Design review of the part built by this model. Coordinates are the model's own, in mm. A direction names the side the tool comes from. Coordinates: 2 decimals unless noted, no trailing zeros. Write each loop counter-clockwise with the first axis right and the second up, starting at its lowest first coordinate (ties: lowest second). Pieces come first, ordered by that corner, then holes. Notation, with made-up numbers: M 66.25,34 L 74.25,34 A19 cw 74.25,53 Z; hole C 83,15.25 d9. An arc over 180 degrees is marked long. Return JSON: item names as keys, results as strings. Group by question number.
```python
from build123d import *

# Parameters (mm, degrees)
F1_DEPTH      = 14
F3_START      = 2
F3_DEPTH      = 9.7
F4_DEPTH      = 1
F4_DEPTH_BACK = 22
F5_START      = 9.5
F5_DEPTH      = 4.5
F6_DEPTH      = 4.5
F8_DEPTH      = 0.5
F9_R          = 1.5933809512
F10_R         = 0.5311269837
F11_T1_DEPTH  = 5.3949137803
F11_T6_ANGLE  = 200.7294916834
F11_T12_ANGLE = 200.7294916834
F12_T1_DEPTH  = 1.2663530932
F12_T3_DEPTH  = 0.9362653772
F12_T5_DEPTH  = 1.4443499817
F12_T7_DEPTH  = 1.4443499817
F12_T9_DEPTH  = 0.9362653772
F12_T11_DEPTH = 1.2663530932
F12_T13_DEPTH = 16.1666666667
F12_T15_DEPTH = 16.1666666667
F12_T17_DEPTH = 15.3725307543
F12_T19_DEPTH = 16.3886999634
F12_T21_DEPTH = 16.3886999634
F12_T23_DEPTH = 15.3725307543
F13_SIZE      = 0.25


# Not quite as in the source:
# - a fillet or chamfer that OpenCascade refuses, or shapes differently, is made with other operations: its cross-section is extruded or revolved along the edge and cut away or added


with BuildPart() as f1:
    # F0 (on Top) → F1 (new body)
    with BuildSketch(Plane.XY):
        Polygon((6.25, 4.4), (0, 4.4), (-6.25, 4.4), (-7.5, 0), (-5.25, -5.4), (-4.395, -5.4), (-4.395, -3.9), (-2.695, -3.9), (-2.695, 0.6), (0, 0.6), (2.695, 0.6), (2.695, -3.9), (4.395, -3.9), (4.395, -5.4), (5.25, -5.4), (7.5, 0), align=None)
    extrude(amount=F1_DEPTH)

    # F2 (on Front) → F3 (cut)
    with BuildSketch(Plane.XZ.offset(F3_START)):
        Polygon((0, 4), (3.875, 4), (3.875, 9), (0, 9), (-3.875, 9), (-3.875, 4), align=None)
    extrude(amount=F3_DEPTH, mode=Mode.SUBTRACT)

    # F2 (on Front) → F4 (cut, two sides)
    with BuildSketch(Plane.XZ) as f4_sk:
        Polygon((-3.875, 1), (0, 1), (3.875, 1), (3.875, 4), (0, 4), (-3.875, 4), align=None)
    extrude(amount=-F4_DEPTH, mode=Mode.SUBTRACT)
    extrude(f4_sk.sketch, amount=F4_DEPTH_BACK, mode=Mode.SUBTRACT)

    # F0 (on Top) → F5 (join)
    with BuildSketch(Plane.XY.offset(F5_START)):
        Polygon((0, -5.4), (4.395, -5.4), (4.395, -3.9), (2.695, -3.9), (2.695, 0.6), (0, 0.6), (-2.695, 0.6), (-2.695, -3.9), (-4.395, -3.9), (-4.395, -5.4), align=None)
    extrude(amount=F5_DEPTH)

    # F6 (add): a face of the model
    f6_faces = [f1.faces().sort_by_distance(p)[0] for p in [
        (0, 0.6, 6.75),
    ]]
    extrude(f6_faces, amount=F6_DEPTH)

    # F7 (on face) → F8 (join)
    with BuildSketch(Plane(origin=(0, 0, 0), x_dir=(1, 0, 0), z_dir=(0, 0, -1))):
        Polygon((4.395, 5.4), (4.395, 4.4), (4.5833333333, 4.4), (6.4426875763, -0.062450183), (5.4945200146, -3.4), (-5.4945200146, -3.4), (-6.4426875763, -0.062450183), (-4.5833333333, 4.4), (-4.395, 4.4), (-4.395, 5.4), (-5.25, 5.4), (-7.5, 0), (-6.25, -4.4), (6.25, -4.4), (7.5, 0), (5.25, 5.4), align=None)
    extrude(amount=F8_DEPTH)

    # F9
    f9_edges = [f1.edges().sort_by_distance(p)[0] for p in [
        (2.695, 0.6, 0.5),
        (-2.695, 0.6, 0.5),
    ]]
    fillet(f9_edges, radius=F9_R)

    # F10
    f10_edges = [f1.edges().sort_by_distance(p)[0] for p in [
        (-3.285, -3.9, 1),
        (3.285, -3.9, 1),
    ]]
    fillet(f10_edges, radius=F10_R)

    # F11: fillet of radius 0.4104163056 on 2 edges, made by hand

    # F11_s2 → F11_t1 (join)
    with BuildSketch(Plane.XZ.offset(-2.026040764)):
        with BuildLine():
            ThreePointArc((3.4645836944, 1), (3.7547918472, 1.1202081528), (3.875, 1.4104163056))
            Line((3.875, 1.4104163056), (3.875, 1))
            Line((3.875, 1), (3.4645836944, 1))
        make_face()
        with BuildLine():
            ThreePointArc((-3.4645836944, 1), (-3.7547918472, 1.1202081528), (-3.875, 1.4104163056))
            Line((-3.875, 1.4104163056), (-3.875, 1))
            Line((-3.875, 1), (-3.4645836944, 1))
        make_face()
    extrude(amount=F11_T1_DEPTH)


with BuildPart() as f11_tool4:
    # F11_s5 → F11_t6 (revolve)
    with BuildSketch(Plane(origin=(0, -2.7915869666, -1.0564952052), x_dir=(1, 0, 0), z_dir=(0, 0.9352619639, 0.3539562952))):
        with BuildLine():
            ThreePointArc((-3.4645836944, -1.0998259262), (-3.7547918472, -0.9796177734), (-3.875, -0.6894096206))
            Line((-3.875, -0.6894096206), (-3.875, -1.0998259262))
            Line((-3.875, -1.0998259262), (-3.4645836944, -1.0998259262))
        make_face()
    revolve(axis=Axis((-3.875, -3.3688730163, 0.4688730163), (-1, 0, 0)), revolution_arc=F11_T6_ANGLE)

    split(bisect_by=Plane.XZ.offset(3.9), keep=Keep.BOTTOM)

    split(bisect_by=Plane.XY, keep=Keep.TOP)


with BuildPart() as f1_1:
    add(f1.part)

    # F11_t3: union F11_tool4
    add(f11_tool4.part)


with BuildPart() as f11_tool10:
    # F11_s11 → F11_t12 (revolve)
    with BuildSketch(Plane(origin=(0, -2.7915869666, -1.0564952052), x_dir=(1, 0, 0), z_dir=(0, 0.9352619639, 0.3539562952))):
        with BuildLine():
            ThreePointArc((3.4645836944, -1.0998259262), (3.7547918472, -0.9796177734), (3.875, -0.6894096206))
            Line((3.875, -0.6894096206), (3.875, -1.0998259262))
            Line((3.875, -1.0998259262), (3.4645836944, -1.0998259262))
        make_face()
    revolve(axis=Axis((3.875, -3.3688730163, 0.4688730163), (-1, 0, 0)), revolution_arc=F11_T12_ANGLE)

    split(bisect_by=Plane.XZ.offset(3.9), keep=Keep.BOTTOM)

    split(bisect_by=Plane.XY, keep=Keep.TOP)


with BuildPart() as f1_2:
    add(f1_1.part)

    # F11_t9: union F11_tool10
    add(f11_tool10.part)

    # F12: fillet of radius 0.5 on 12 edges, made by hand

    # F12_s2 → F12_t1 (join)
    with BuildSketch(Plane.XY.offset(-0.5)):
        with BuildLine():
            ThreePointArc((-4.395, -4.4), (-4.5790190998, -4.2919632329), (-4.7012338092, -4.1170388579))
            Line((-4.7012338092, -4.1170388579), (-4.5833333333, -4.4))
            Line((-4.5833333333, -4.4), (-4.395, -4.4))
        make_face()
    extrude(amount=F12_T1_DEPTH)

    # F12_s4 → F12_t3 (join)
    with BuildSketch(Plane.XY.offset(-0.5)):
        with BuildLine():
            ThreePointArc((-6.3755698259, -0.0986324178), (-6.4131614706, 0.0641941432), (-6.3949990431, 0.2303138196))
            Line((-6.3949990431, 0.2303138196), (-6.4426875763, 0.062450183))
            Line((-6.4426875763, 0.062450183), (-6.3755698259, -0.0986324178))
        make_face()
    extrude(amount=F12_T3_DEPTH)

    # F12_s6 → F12_t5 (join)
    with BuildSketch(Plane.XY.offset(-0.5)):
        with BuildLine():
            ThreePointArc((-5.5977477007, 3.0366385451), (-5.4181773738, 3.2989481624), (-5.1167800219, 3.4))
            Line((-5.1167800219, 3.4), (-5.4945200146, 3.4))
            Line((-5.4945200146, 3.4), (-5.5977477007, 3.0366385451))
        make_face()
    extrude(amount=F12_T5_DEPTH)

    # F12_s8 → F12_t7 (join)
    with BuildSketch(Plane.XY.offset(-0.5)):
        with BuildLine():
            ThreePointArc((5.1167800219, 3.4), (5.4181773738, 3.2989481624), (5.5977477007, 3.0366385451))
            Line((5.5977477007, 3.0366385451), (5.4945200146, 3.4))
            Line((5.4945200146, 3.4), (5.1167800219, 3.4))
        make_face()
    extrude(amount=F12_T7_DEPTH)

    # F12_s10 → F12_t9 (join)
    with BuildSketch(Plane.XY.offset(-0.5)):
        with BuildLine():
            ThreePointArc((6.3949990431, 0.2303138196), (6.4131614706, 0.0641941432), (6.3755698259, -0.0986324178))
            Line((6.3755698259, -0.0986324178), (6.4426875763, 0.062450183))
            Line((6.4426875763, 0.062450183), (6.3949990431, 0.2303138196))
        make_face()
    extrude(amount=F12_T9_DEPTH)

    # F12_s12 → F12_t11 (join)
    with BuildSketch(Plane.XY.offset(-0.5)):
        with BuildLine():
            ThreePointArc((4.7012338092, -4.1170388579), (4.5790190998, -4.2919632329), (4.395, -4.4))
            Line((4.395, -4.4), (4.5833333333, -4.4))
            Line((4.5833333333, -4.4), (4.7012338092, -4.1170388579))
        make_face()
    extrude(amount=F12_T11_DEPTH)

    # F12_s14 → F12_t13 (cut)
    with BuildSketch(Plane.XY.offset(-1.3333333333)):
        with BuildLine():
            ThreePointArc((-4.9166666667, -5.4), (-5.1940167648, -5.3160251472), (-5.3782051282, -5.0923076923))
            Line((-5.3782051282, -5.0923076923), (-5.25, -5.4))
            Line((-5.25, -5.4), (-4.9166666667, -5.4))
        make_face()
    extrude(amount=F12_T13_DEPTH, mode=Mode.SUBTRACT)

    # F12_s16 → F12_t15 (cut)
    with BuildSketch(Plane.XY.offset(-1.3333333333)):
        with BuildLine():
            ThreePointArc((4.9166666667, -5.4), (5.1940167648, -5.3160251472), (5.3782051282, -5.0923076923))
            Line((5.3782051282, -5.0923076923), (5.25, -5.4))
            Line((5.25, -5.4), (4.9166666667, -5.4))
        make_face()
    extrude(amount=F12_T15_DEPTH, mode=Mode.SUBTRACT)

    # F12_s18 → F12_t17 (cut)
    with BuildSketch(Plane.XY.offset(-0.9362653772)):
        with BuildLine():
            ThreePointArc((7.4328822497, -0.1610826008), (7.4704738943, 0.0017439601), (7.4523114669, 0.1678636366))
            Line((7.4523114669, 0.1678636366), (7.5, 0))
            Line((7.5, 0), (7.4328822497, -0.1610826008))
        make_face()
    extrude(amount=F12_T17_DEPTH, mode=Mode.SUBTRACT)

    # F12_s20 → F12_t19 (cut)
    with BuildSketch(Plane.XY.offset(-1.4443499817)):
        with BuildLine():
            ThreePointArc((6.3532276861, 4.0366385451), (6.1736573592, 4.2989481624), (5.8722600073, 4.4))
            Line((5.8722600073, 4.4), (6.25, 4.4))
            Line((6.25, 4.4), (6.3532276861, 4.0366385451))
        make_face()
    extrude(amount=F12_T19_DEPTH, mode=Mode.SUBTRACT)

    # F12_s22 → F12_t21 (cut)
    with BuildSketch(Plane.XY.offset(-1.4443499817)):
        with BuildLine():
            ThreePointArc((-5.8722600073, 4.4), (-6.1736573592, 4.2989481624), (-6.3532276861, 4.0366385451))
            Line((-6.3532276861, 4.0366385451), (-6.25, 4.4))
            Line((-6.25, 4.4), (-5.8722600073, 4.4))
        make_face()
    extrude(amount=F12_T21_DEPTH, mode=Mode.SUBTRACT)

    # F12_s24 → F12_t23 (cut)
    with BuildSketch(Plane.XY.offset(-0.9362653772)):
        with BuildLine():
            ThreePointArc((-7.4523114669, 0.1678636366), (-7.4704738943, 0.0017439601), (-7.4328822497, -0.1610826008))
            Line((-7.4328822497, -0.1610826008), (-7.5, 0))
            Line((-7.5, 0), (-7.4523114669, 0.1678636366))
        make_face()
    extrude(amount=F12_T23_DEPTH, mode=Mode.SUBTRACT)

    # F13
    f13_edges = [f1_2.edges().sort_by_distance(p)[0] for p in [
        (-5.996373, 1.633476, 0),
        (-5.418177, 3.298948, 0),
        (-6.413161, 0.064194, 0),
        (-5.538402, -2.107836, 0),
        (-4.579019, -4.291963, 0),
        (4.579019, -4.291963, 0),
        (5.538402, -2.107836, 0),
        (6.413161, 0.064194, 0),
        (5.996373, 1.633476, 0),
        (5.418177, 3.298948, 0),
        (0, 3.4, 0),
    ]]
    chamfer(f13_edges, length=F13_SIZE)


solid = f1_2.part
```
Item 1: The part is to be moulded in two halves that separate along X. For faces 1 (the cylindrical face through (-2.216, 0.146, 0.507)), 2 (the flat face through (-1, 4, -0.5)), 3 (the flat face through (6.895, 2.129, 6.852)), say which applies: pulls with the +X half, pulls with the -X half, needs draft (parallel to the pull), parting line crosses it, or undercut.
Item 2: For pin 1 (1.3 mm diameter, centred on x = -3.5, z = 7.5, fed in from -Y); pin 2 (0.9 mm diameter, centred on x = -3, y = -2.5, fed in from -Z); pin 3 (1.5 mm diameter, centred on y = 2.5, z = 4.5, fed in from +X), all flat-tipped, find the tip position at first contact; note any pin that passes through.
Item 3: Add section D-D (x = -3). Write out the cut boundary in (y, z).
Item 4: Add section C-C (y = -1.5). Write out the cut boundary in (x, z) (3 decimals), plus the area to 3 significant figures.
Item 5: Add section A-A (x = -0.75). Write out the cut boundary in (y, z), plus the area to 3 significant figures.
Item 6: Machinability: for faces 4 (the flat face through (2.695, -3, 6)), 5 (the flat face through (0, 0.6, 0.5)), 6 (the flat face through (1, -5.4, 10)), which of the approach directions +Z, -Z, +X, -X, +Y, -Y give a long, thin tool a straight path to every point of the face, cutting with its end or side? Answer none if there is none.
Item 7: For line 1 (Z direction, x = 2, y = 0.75); line 2 (Z direction, x = -0.25, y = 0.5); line 3 (Z direction, x = 2, y = -4), list the stretches that pass through material, from the lowest coordinate up.
Item 8: Add section B-B (z = 9.25). Write out the cut boundary in (x, y) (3 decimals).
Geometry check:
{
 "1": {"face 1": "undercut", "face 2": "needs draft", "face 3": "pulls with the +X half"},
 "2": {"pin 1": "y = -3.9", "pin 2": "z = 0", "pin 3": "x = 7"},
 "3": {"outline": "M -5.4,9.5 L -3.9,9.5 L -3.9,9 L -2,9 L -2,4 L 1,4 L 1,1 L -3.37,1 A0.53 ccw -3.9,0.47 L -3.9,0 L 3.15,0 L 3.4,-0.25 L 3.4,-0.5 L 4.4,-0.5 L 4.4,14 L -5.4,14 Z"},
 "4": {"outline": "M -6.875,-0.5 L -5.792,-0.5 L -5.792,-0.25 L -5.521,0 L -2.695,0 L -2.695,1 L -3.465,1 A0.41 cw -3.875,1.41 L -3.875,4 L 3.875,4 L 3.875,1.41 A0.41 cw 3.465,1 L 2.695,1 L 2.695,0 L 5.521,0 L 5.792,-0.25 L 5.792,-0.5 L 6.875,-0.5 L 6.875,14 L -6.875,14 Z", "area": "165 mm^2"},
 "5": {"outline": "M -5.4,9.5 L -3.9,9.5 L -3.9,4 L 1,4 L 1,1 L 0.6,1 L 0.6,0 L 3.15,0 L 3.4,-0.25 L 3.4,-0.5 L 4.4,-0.5 L 4.4,14 L -5.4,14 Z", "area": "104 mm^2"},
 "6": {"face 4": "-Y", "face 5": "-Z, -Y", "face 6": "+Z, -Z, +X, -X, -Y"},
 "7": {"line 1": "0 to 1, 4 to 14", "line 2": "4 to 14", "line 3": "9.5 to 14"},
 "8": {"outline": "M -7.452,0.168 A0.5 ccw -7.433,-0.161 L -5.378,-5.092 A0.5 ccw -4.917,-5.4 L -4.395,-5.4 L -4.395,-3.9 L 4.395,-3.9 L 4.395,-5.4 L 4.917,-5.4 A0.5 ccw 5.378,-5.092 L 7.433,-0.161 A0.5 ccw 7.452,0.168 L 6.353,4.037 A0.5 ccw 5.872,4.4 L -5.872,4.4 A0.5 ccw -6.353,4.037 Z"}
}
